Geometry: see drawing. Coordinates: mm, zero at the bounding-box minimum. A direction names the side the tool comes from. Give positions to 0.01 mm unless a question says otherwise; leave off trailing zeros. Loops run counter-clockwise (first coordinate to the right, second up) from the corner with the lowest first, then second, coordinate; pieces in that order, holes last. Notation, with made-up numbers: (51, -9.75) - (107, -9.75) arc R16 ccw to (107, 6.25) - close; hole circle Ø1 at (49, 9). An arc over 180 degrees is marked (long way). Use CSV: the item, a comma, the result in double quotes. Start each with the question number.
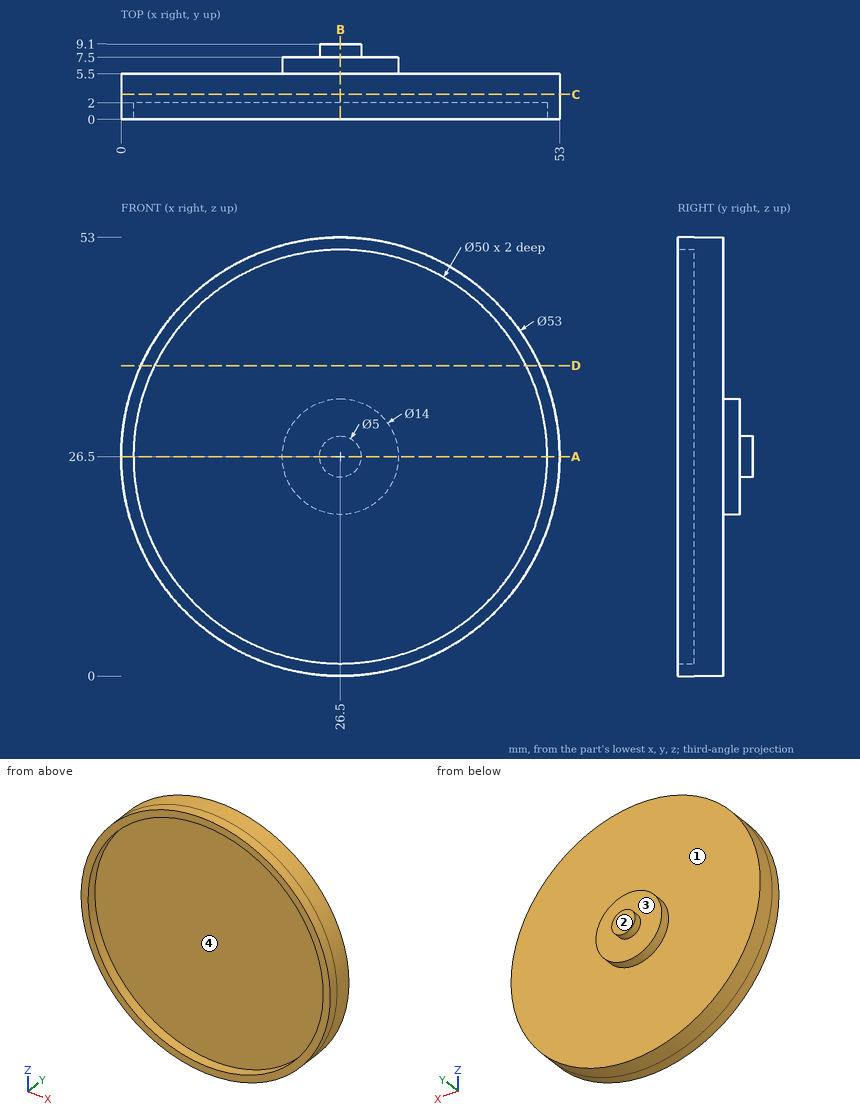
Item 1: Section D-D (z = 37.5). Output: boundary loops of the cut face in (x, y).
Item 2: Section C-C (y = 3). Output: boundary loops of the cut face in (x, z), plus the area to 3 significant figures.
Item 3: Section B-B (x = 26.5). Output: boundary loops of the cut face in (y, z), plus the area to 4 significant figures.
Item 4: Ray query, probe 1 along X at (y, z) = (1.6, 26.5); probe 2 along Y at (x, z) = (37, 16.5); probe 3 along Y at (x, z) = (32.5, 28). Return the intervals inside material, ascending.
Item 5: Mould query, pull axis Z, two halves, no side actions, for the marked faces 3 and 4. Classes: pulls with the +Z half, pulls with the -Z half, needs draft (parallel to the pull), parting line crosses it, or undercut.
Item 6: Pin query (flat end, axial travel): pin 1 Ø3 at (x, y) = (47.5, 1.5) entering from +Z; pin 2 Ø3 at (x, y) = (30, 2.5) entering from +Z; pin 3 Ø3 at (x, y) = (41, 4) entering from -Z; pin 4 Ø4 at (x, z) = (24.5, 23.5) entering from +Y. Return the tip coordinate at first contact, or that it passes through.
Item 7: Section A-A (z = 26.5). Output: boundary loops of the cut face in (x, y).
Item 8: Reachability of the marked faces 1 and 2 from +Z, -Z, +X, -X, +Y, -Y: full face, straight path, thin tool, end or side. Return the list, or none.
Outcome:
1,outline,"(2.39, 0) - (4.05, 0) - (4.05, 2) - (48.95, 2) - (48.95, 0) - (50.61, 0) - (50.61, 5.5) - (2.39, 5.5) - close"
2,outline,"circle Ø53 at (26.5, 26.5)"
2,area,"2,210 mm2"
3,outline,"(0, 0) - (5.5, 0) - (5.5, 19.5) - (7.5, 19.5) - (7.5, 24) - (9.1, 24) - (9.1, 29) - (7.5, 29) - (7.5, 33.5) - (5.5, 33.5) - (5.5, 53) - (0, 53) - (0, 51.5) - (2, 51.5) - (2, 1.5) - (0, 1.5) - close"
3,area,"227.5 mm2"
4,probe 1,"x = 0 to 1.5, 51.5 to 53"
4,probe 2,"y = 2 to 5.5"
4,probe 3,"y = 2 to 7.5"
5,face 3,"needs draft"
5,face 4,"undercut"
6,pin 1,"stops at z = 44.44"
6,pin 2,"stops at z = 52.92"
6,pin 3,"stops at z = 3.41"
6,pin 4,"stops at y = 9.1"
7,outline,"(0, 0) - (1.5, 0) - (1.5, 2) - (51.5, 2) - (51.5, 0) - (53, 0) - (53, 5.5) - (33.5, 5.5) - (33.5, 7.5) - (29, 7.5) - (29, 9.1) - (24, 9.1) - (24, 7.5) - (19.5, 7.5) - (19.5, 5.5) - (0, 5.5) - close"
8,face 1,"+Y"
8,face 2,"+Z, -Z, +X, -X, +Y"
